Input: part model. Units: mm. Frame: model coordinates. Face numbers are marked on the shaded views. A direction names the side the tool comes from. Give positions to 0.01 mm unless a question says otherwise; leave off trailing zeros. Write each loop counter-clockwise with the first axis right and the second up, starting at its lowest first coordinate (ties: lowest second). Pieces come first, ordered by that corner, then holes. Notation, with made-up numbers: (68, 35) - (116, 35) arc R12 cw to (116, 43) - close; hole circle Ø6 at (7.5, -11). An arc over 180 degrees is marked (long way). Use a Markdown table: item, result. Add a question column.
1. Pin query (flat end, axial travel): pin 1 (4 mm diameter, centred on y = 10.5, z = 1.5, fed in from +X); pin 2 (5 mm diameter, centred on x = -4.5, y = 6, fed in from +Z); pin 3 (1.5 mm diameter, centred on x = -2, y = 10.5, fed in from +Z); pin 4 (2 mm diameter, centred on x = -4.5, y = 11, fed in from -Z). Return the tip coordinate at first contact, or that it passes through.
2. Set-up query: the marked faces 1 and 2. Return all of +Z, -Z, +X, -X, +Y, -Y with unobstructed straight access to the full face (end or side cutting, diameter ignored); none if empty.
3. Section query B-B, the plane x = 1. Count the separate pieces of the cut face and the enclosed holes in it, plus the area to 3 significant figures.
4. Material intervals for probe 1 along Z at (x, y) = (4, 4); probe 2 along X at (y, z) = (7.25, 1.5); probe 3 along X at (y, z) = (9.5, 2.75), sorted ascending.
5. Section query C-C, the plane y = 5. Return loops of the section in (x, z), plus the area to 3 significant figures.
6. Section query D-D, the plane y = 2.5. Return loops of the section in (x, z).
7. Section query A-A, the plane y = 7. Return loops of the section in (x, z), plus the area to 3 significant figures.
8. Mould query, pull axis X, two halves, no side actions, for the marked faces 3, 4 and 5. Classes: released by +X, released by -X, zero draft, split by the parting line, or undercut.
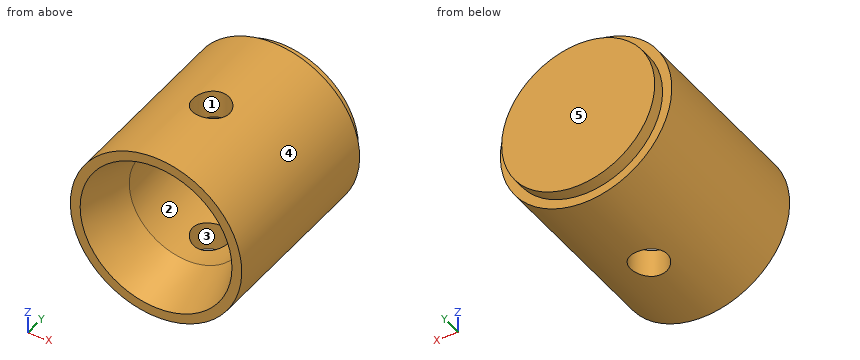
```python
from build123d import *

# Parameters (mm, degrees)
SKETCH1_R               = 7
BOSS_EXTRUDE1_DEPTH     = 16
CUT_EXTRUDE1_DEPTH      = 19.814887722
CUT_EXTRUDE1_DEPTH_BACK = 19.814887722
SKETCH2_R               = 1.5
SKETCH3_R               = 4.75
CUT_EXTRUDE2_DEPTH      = 11
CUT_EXTRUDE3_START      = -1
SKETCH6_R               = 7
SKETCH6_R_2             = 6.25
CUT_EXTRUDE3_DEPTH      = 1


with BuildPart() as part:
    # Sketch1 → Boss-Extrude1 (new body)
    with BuildSketch(Plane(origin=(0, 0, 0), x_dir=(1, 0, 0), z_dir=(0, 1, 0))):
        with Locations(Location((0, 0, 0), (0, 0, 270))):
            Circle(SKETCH1_R)
    extrude(amount=BOSS_EXTRUDE1_DEPTH)

    # Sketch2 → Cut-Extrude1 (cut, two sides: drawn at the far end of the back side and taken through both)
    with BuildSketch(Plane.XY.offset(-CUT_EXTRUDE1_DEPTH_BACK)):
        with Locations(Location((0, 7, 0), (0, 0, 90.000000049))):
            Circle(SKETCH2_R)
    extrude(amount=CUT_EXTRUDE1_DEPTH + CUT_EXTRUDE1_DEPTH_BACK, mode=Mode.SUBTRACT)

    # Sketch3 → Cut-Extrude2 (cut)
    with BuildSketch(Plane.XZ):
        with Locations(Location((0, 0, 0), (0, 0, 270))):
            Circle(SKETCH3_R)
    extrude(amount=-CUT_EXTRUDE2_DEPTH, mode=Mode.SUBTRACT)

    # Sketch4 → Cut-Revolve1 (revolve, cut)
    with BuildSketch(Plane.XY, mode=Mode.PRIVATE) as cut_revolve1_sk:
        Polygon((0, 11), (0, 13.85408794), (4.75, 11), align=None)
    revolve(cut_revolve1_sk.sketch.rotate(Axis((0, 11, 0), (0, 1, 0)), 90), axis=Axis((0, 11, 0), (0, 1, 0)), mode=Mode.SUBTRACT)

    # Sketch5 → Cut-Revolve2 (revolve, cut)
    with BuildSketch(Plane.XY, mode=Mode.PRIVATE) as cut_revolve2_sk:
        Polygon((4.75, 0), (4.75, 3.983842258), (6.2, 0), align=None)
    revolve(cut_revolve2_sk.sketch.rotate(Axis((0, 0, 0), (0, 1, 0)), 90), axis=Axis((0, 0, 0), (0, 1, 0)), mode=Mode.SUBTRACT)

    # Sketch6 → Cut-Extrude3 (cut)
    with BuildSketch(Plane(origin=(0, 16, 0), x_dir=(1, 0, 0), z_dir=(0, 1, 0)).offset(CUT_EXTRUDE3_START)):
        with Locations(Location((0, 0, 0), (0, 0, 270))):
            Circle(SKETCH6_R)
        with Locations(Location((0, 0, 0), (0, 0, 270))):
            Circle(SKETCH6_R_2, mode=Mode.SUBTRACT)
    extrude(amount=CUT_EXTRUDE3_DEPTH, mode=Mode.SUBTRACT)


solid = part.part
```
Result sheet:
| question | item | result |
|---|---|---|
| 1 | pin 1 | stops at x = 7 |
| 1 | pin 2 | stops at z = 6.71 |
| 1 | pin 3 | stops at z = 6.89 |
| 1 | pin 4 | stops at z = -6.06 |
| 2 | face 1 | +Z, -Z |
| 2 | face 2 | -Y |
| 3 | separate pieces | 3 |
| 3 | enclosed holes | 0 |
| 3 | area | 90.0 mm² |
| 4 | probe 1 | z = -5.74 to -2.56, 2.56 to 5.74 |
| 4 | probe 2 | x = -6.84 to -4.51, 4.51 to 6.84 |
| 4 | probe 3 | x = -6.44 to -3.87, 3.87 to 6.44 |
| 5 | outline | circle Ø14 at (0, 0); hole circle Ø9.5 at (0, 0) |
| 5 | area | 83.1 mm² |
| 6 | outline | circle Ø14 at (0, 0); hole circle Ø10.58 at (0, 0) |
| 7 | outline | (-1.5, -6.84) - (-1.5, -4.51) arc R4.75 cw to (-1.5, 4.51) - (-1.5, 6.84) arc R7 ccw to start; (1.5, -6.84) arc R7 ccw to (1.5, 6.84) - (1.5, 4.51) arc R4.75 cw to (1.5, -4.51) - close |
| 7 | area | 69.4 mm² |
| 8 | face 3 | undercut |
| 8 | face 4 | split by the parting line |
| 8 | face 5 | zero draft |
